```python
from build123d import *

# Parameters (mm, degrees)
SKETCH1_W               = 80
SKETCH1_H               = 150
SKETCH1_W_2             = 70
SKETCH1_H_2             = 140
EXTRUDE_THIN1_DEPTH     = 25
CUT_EXTRUDE1_DEPTH      = 1
CUT_EXTRUDE1_DEPTH_BACK = 81
FILLET1_R               = 20
SKETCH3_R               = 3
SKETCH3_R_2             = 1.5
SKETCH3_R_3             = 6
CUT_EXTRUDE2_DEPTH      = 1.0000001
CUT_EXTRUDE2_DEPTH_BACK = 81.0000001
SKETCH5_R               = 1.5
BOSS_EXTRUDE1_DEPTH     = 4
SKETCH6_R               = 3
CUT_EXTRUDE3_DEPTH      = 10


with BuildPart() as part:
    # Sketch1 → Extrude-Thin1 (new body, symmetric)
    with BuildSketch(Plane.XY):
        Rectangle(SKETCH1_W, SKETCH1_H)
        Rectangle(SKETCH1_W_2, SKETCH1_H_2, mode=Mode.SUBTRACT)
    extrude(amount=EXTRUDE_THIN1_DEPTH, both=True)

    # Sketch2 → Cut-Extrude1 (cut, two sides)
    with BuildSketch(Plane(origin=(40, 0, 0), x_dir=(0, 0, -1), z_dir=(1, 0, 0))) as cut_extrude1_sk:
        with BuildLine():
            Line((-25, -15.384333338), (-10, -15.384333338))
            ThreePointArc((-10, -15.384333338), (-2.928932188, -12.45540115), (0, -5.384333338))
            Line((0, -5.384333338), (0, 75))
            Line((0, 75), (-25, 75))
            Line((-25, 75), (-25, -15.384333338))
        make_face()
    extrude(amount=CUT_EXTRUDE1_DEPTH, mode=Mode.SUBTRACT)
    extrude(cut_extrude1_sk.sketch, amount=-CUT_EXTRUDE1_DEPTH_BACK, mode=Mode.SUBTRACT)

    # Fillet1
    fillet1_edges = [part.edges().sort_by_distance(p)[0] for p in [
        (-37.5, -15.384333338, 25),
        (37.5, -15.384333338, 25),
    ]]
    fillet(fillet1_edges, radius=FILLET1_R)

    # Sketch3 → Cut-Extrude2 (cut, two sides)
    with BuildSketch(Plane(origin=(40, 0, 0), x_dir=(0, 0, -1), z_dir=(1, 0, 0))) as cut_extrude2_sk:
        with Locations((12.5, 0.5)):
            Circle(SKETCH3_R)
        with Locations((0, -24.070063275)):
            Circle(SKETCH3_R_2)
        with Locations((12.817814142, -46.271168612)):
            Circle(SKETCH3_R_2)
        with Locations((0, -45.523799356)):
            Circle(SKETCH3_R_3)
        with Locations((-12.817814142, -46.271168612)):
            Circle(SKETCH3_R_2)
        with BuildLine():
            Line((16, 60), (16, 15.5))
            ThreePointArc((16, 15.5), (12.5, 12), (9, 15.5))
            Line((9, 15.5), (9, 60))
            ThreePointArc((9, 60), (12.5, 63.5), (16, 60))
        make_face()
    extrude(amount=CUT_EXTRUDE2_DEPTH, mode=Mode.SUBTRACT)
    extrude(cut_extrude2_sk.sketch, amount=-CUT_EXTRUDE2_DEPTH_BACK, mode=Mode.SUBTRACT)

    # Sketch5 → Boss-Extrude1 (add)
    with BuildSketch(Plane.XZ.offset(-70)):
        with Locations((0, -12.5)):
            Circle(SKETCH5_R)
    extrude(amount=BOSS_EXTRUDE1_DEPTH)

    # Sketch6 → Cut-Extrude3 (cut)
    with BuildSketch(Plane(origin=(0, -70, 0), x_dir=(1, 0, 0), z_dir=(0, 1, 0))):
        with Locations((20, 0)):
            Circle(SKETCH6_R)
        with Locations((-20, 0)):
            Circle(SKETCH6_R)
    extrude(amount=-CUT_EXTRUDE3_DEPTH, mode=Mode.SUBTRACT)


solid = part.part
```
Build history of the part. All positions in model axes, mm. A direction names the side the tool comes from. Round coordinates to 2 decimals unless told otherwise and drop trailing zeros. Write each loop counter-clockwise with the first axis right and the second up, starting at its lowest first coordinate (ties: lowest second). Pieces come first, ordered by that corner, then holes.
1) Drill centre lines: probe 1 along Y at (x, z) = (-27, -1.5); probe 2 along X at (y, z) = (-71.95, 0); probe 3 along X at (y, z) = (-57.5, 14). Where is each one in solid material? Low to high.
2) Band-saw the part on D-D, the plane z = -4.5. List the corners of the cut face in (x, y).
3) Band-saw the part on C-C, the plane x = 0. List the corners of the cut face in (y, z), and give its area (3 significant figures).
4) Mould opens along X. For faces 6 (the flat face through (3, -71, 25)), 7 (the flat face through (40, -18, -5)), 8 (the flat face through (0, -70, 0)) say: +X half, -X half, draft (parallel to the pull), parting line (faces both ways), or undercut.
5) Band-saw the part on A-A, the plane x = -20. List the corners of the cut face in (y, z), and give its area (3 significant figures).
6) 3-axis set-ups, long thin cutter, end or side, ignore diameter. For faces 1 (the flat face through (-35, -17, -5)), 2 (the flat face through (-5.7, 70.3, 0)), 3 (the flat face through (-36, 6, -25)), 4 (the cylindrical face through (-23, -72, 0)), 5 (the flat face through (38, 38, -16)): which of +Z, -Z, +X, -X, +Y, -Y reach the whole face in a straight line?
7) Band-saw the part on B-B, the plane y = 22. List the corners of the cut face in (x, z).
8) Pin check, flat tips, straight feed: pin 1 (1.5 mm diameter, centred on x = 37.5, y = 36.5, fed in from +Z); pin 2 (6 mm diameter, centred on x = -16, z = 4.5, fed in from +Y). Stop position of each tip, or through.
Ans:
1. probe 1: y = -75 to -70, 70 to 75
1. probe 2: x = -40 to -23, -17 to 17, 23 to 40
1. probe 3: x = -40 to -35, 35 to 40
2. outline: (-40, -75) - (40, -75) - (40, -49.49) - (35, -49.49) - (35, -70) - (-35, -70) - (-35, -49.49) - (-40, -49.49) - close; (-40, -41.56) - (-35, -41.56) - (-35, 70) - (35, 70) - (35, -41.56) - (40, -41.56) - (40, 75) - (-40, 75) - close
3. outline: (-75, -25) - (-70, -25) - (-70, 25) - (-75, 25) - close; (66, -14) - (70, -14) - (70, -25) - (75, -25) - (75, 0) - (70, 0) - (70, -11) - (66, -11) - close
3. area: 387 mm2
4. face 6: draft
4. face 7: +X half
4. face 8: undercut
5. outline: (-75, -25) - (-70, -25) - (-70, -3) - (-75, -3) - close; (-75, 3) - (-70, 3) - (-70, 25) - (-75, 25) - close; (70, -25) - (75, -25) - (75, 0) - (70, 0) - close
5. area: 345 mm2
6. face 1: +Z, -Z
6. face 2: +Z, +X, -X, +Y
6. face 3: -Z, +X, -X, +Y, -Y
6. face 4: -Y
6. face 5: +X, -X
7. outline: (-40, -25) - (-35, -25) - (-35, -16) - (-40, -16) - close; (-40, -9) - (-35, -9) - (-35, 0) - (-40, 0) - close; (35, -25) - (40, -25) - (40, -16) - (35, -16) - close; (35, -9) - (40, -9) - (40, 0) - (35, 0) - close
8. pin 1: stops at z = 0
8. pin 2: stops at y = -70
